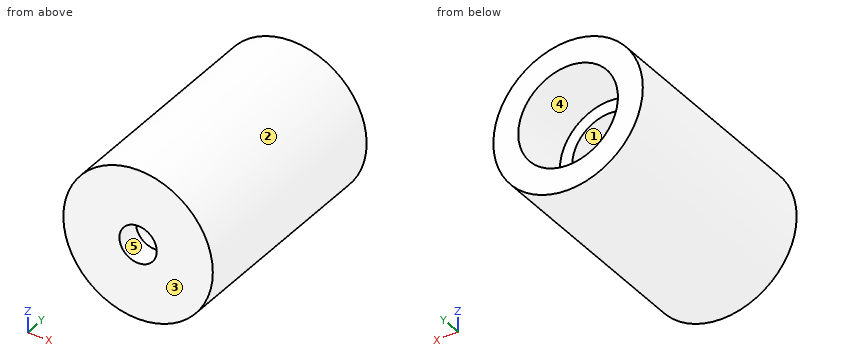
```python
from build123d import *

# Parameters (mm, degrees)
SKETCH2_R           = 6
BOSS_EXTRUDE2_DEPTH = 18.5
SKETCH3_R           = 4
CUT_EXTRUDE1_DEPTH  = 16.5
CUT_EXTRUDE2_REACH  = 4
SKETCH4_R           = 1.5
SKETCH5_R           = 4
SKETCH5_R_2         = 3
BOSS_EXTRUDE3_DEPTH = 11.5


with BuildPart() as part:
    # Sketch2 → Boss-Extrude2 (new body)
    with BuildSketch(Plane(origin=(0, 0, 0), x_dir=(1, 0, 0), z_dir=(0, 1, 0))):
        Circle(SKETCH2_R)
    extrude(amount=BOSS_EXTRUDE2_DEPTH)

    # Sketch3 → Cut-Extrude1 (cut)
    with BuildSketch(Plane(origin=(0, 18.5, 0), x_dir=(1, 0, 0), z_dir=(0, 1, 0))):
        Circle(SKETCH3_R)
    extrude(amount=-CUT_EXTRUDE1_DEPTH, mode=Mode.SUBTRACT)

    # Sketch4 → Cut-Extrude2 (cut, up to next)
    with BuildSketch(Plane(origin=(0, 2, 0), x_dir=(1, 0, 0), z_dir=(0, 1, 0)), mode=Mode.PRIVATE) as cut_extrude2_sk1:
        Circle(SKETCH4_R)
    cut_extrude2_tool1 = extrude(cut_extrude2_sk1.sketch, amount=-CUT_EXTRUDE2_REACH, mode=Mode.PRIVATE) & part.part
    add(cut_extrude2_tool1.solids().sort_by_distance((0, 2, 0))[0], mode=Mode.SUBTRACT)

    # Sketch5 → Boss-Extrude3 (add)
    with BuildSketch(Plane(origin=(0, 2, 0), x_dir=(1, 0, 0), z_dir=(0, 1, 0))):
        Circle(SKETCH5_R)
        Circle(SKETCH5_R_2, mode=Mode.SUBTRACT)
    extrude(amount=BOSS_EXTRUDE3_DEPTH)


solid = part.part
```
CAD build for the part. Positions are in the model's coordinates, mm. Face numbers are marked on the shaded views. A direction names the side the tool comes from. Coordinates: 2 decimals unless noted, no trailing zeros. Order: outer loops, then holes, each group sorted by start corner. A loop starts at its lowest first (then second) coordinate and runs counter-clockwise, first axis right, second up. Notation, with made-up numbers: (5.25, 38.25) - (35.25, 38.25) arc R13 ccw to (35.25, 60.25) - close; hole circle Ø4 at (-25.75, 66.25). An arc over 180 degrees is marked (long way). Use a Markdown table: item, result. Add a question column.
(1) Flat gauge pins, fed straight in: pin 1 (4 mm diameter, centred on x = 0, z = 0, fed in from +Y); pin 2 (2 mm diameter, centred on x = -3.5, y = 2, fed in from -Z); pin 3 (1.5 mm diameter, centred on x = 4.5, y = 6, fed in from -Z). Where does each tip first touch, or does it go through?
(2) Saw through at D-D (x = 3.25). Give the cut face in (y, z).
(3) Saw through at C-C (y = 13). Give the cut face in (x, z), then the cut area to 3 significant figures.
(4) Saw through at A-A (z = 0). Give the cut face in (x, y).
(5) Which spindle directions (+Z, -Z, +X, -X, +Y, -Y) get a long thin tool onto all of the face, cutting with end or side? Do the marked faces 4 and 5. Say none if no direction does.
(6) Drill centre lines: line 1 along Z through (x, y) = (0, 14.85); line 2 along X through (y, z) = (10.75, 0); line 3 along X through (y, z) = (0.5, 0). Where is each one in solid material? Low to high. Write a range as [from, to].
(7) Pull direction Z, two halves, no side cores. Call the marked faces 1, 2 and 3: +Z half, -Z half, draft (parallel to the pull), parting line (faces both ways), or undercut.
(8) Saw through at B-B (x = 0). Give the cut face in (y, z).
Solved:
| question | item | result |
|---|---|---|
| 1 | pin 1 | stops at y = 2 |
| 1 | pin 2 | stops at z = -5.45 |
| 1 | pin 3 | stops at z = -4.68 |
| 2 | outline | (0, -5.04) - (18.5, -5.04) - (18.5, -2.33) - (13.5, -2.33) - (13.5, 2.33) - (18.5, 2.33) - (18.5, 5.04) - (0, 5.04) - close |
| 3 | outline | circle Ø12 at (0, 0); hole circle Ø6 at (0, 0) |
| 3 | area | 84.8 mm² |
| 4 | outline | (-6, 0) - (-1.5, 0) - (-1.5, 2) - (-3, 2) - (-3, 13.5) - (-4, 13.5) - (-4, 18.5) - (-6, 18.5) - close; (1.5, 0) - (6, 0) - (6, 18.5) - (4, 18.5) - (4, 13.5) - (3, 13.5) - (3, 2) - (1.5, 2) - close |
| 5 | face 4 | +Y |
| 5 | face 5 | +Y, -Y |
| 6 | line 1 | z = [-6, -4], [4, 6] |
| 6 | line 2 | x = [-6, -3], [3, 6] |
| 6 | line 3 | x = [-6, -1.5], [1.5, 6] |
| 7 | face 1 | undercut |
| 7 | face 2 | parting line |
| 7 | face 3 | draft |
| 8 | outline | (0, -6) - (18.5, -6) - (18.5, -4) - (13.5, -4) - (13.5, -3) - (2, -3) - (2, -1.5) - (0, -1.5) - close; (0, 1.5) - (2, 1.5) - (2, 3) - (13.5, 3) - (13.5, 4) - (18.5, 4) - (18.5, 6) - (0, 6) - close |
